CAD build for the part. Positions are in the model's coordinates, mm. A direction names the side the tool comes from. Give positions to 0.01 mm unless a question says otherwise; leave off trailing zeros. Order: outer loops, then holes, each group sorted by start corner. A loop starts at its lowest first (then second) coordinate and runs counter-clockwise, first axis right, second up.
Item 1: Band-saw the part on D-D on y = -13. Give the cut face in (x, z).
Item 2: Flat gauge pins, fed straight in: P1, Ø1.2, axis at y = -10.5, z = 2.5, coming from the -X side; P2, Ø2, axis at y = -8.5, z = 1.5, coming from the +X side; P3, Ø1.5, axis at x = -5, z = 1.5, coming from the -Y side. Where does each tip first touch, or does it go through?
Item 3: Band-saw the part on A-A on z = 0.9. Give the cut face in (x, y).
Item 4: Which spindle directions (+Z, -Z, +X, -X, +Y, -Y) get a long thin tool onto all of the face, cutting with end or side? Do faces 1 (the flat face through (2, -4, 0)), 2 (the flat face through (-2, -12, 2)), 3 (the flat face through (-2, 3, 2)). Say none if no direction does.
Item 5: Wall check: L1, parallel to X at y = -2, z = 2.55; L2, parallel to X at y = 5.25, z = 3.7; L3, parallel to X at y = -10, z = 3.4. Give the ranges that are in metal, low to high.
Item 6: Band-saw the part on B-B on y = 1. Give the cut face in (x, z).
Item 7: Two-plate mould, pull along X, no slides. Class faces 4 (the cylindrical face through (0, -5, 2)), 5 (the cylindrical face through (-8.1, -0.1, 2)), 6 (the flat face through (2, -12, 2)): released by +X, released by -X, zero draft, split by the parting line, or undercut.
Item 8: Band-saw the part on C-C on x = 0. Give the cut face in (y, z).
```python
from build123d import *

# Parameters (mm, degrees)
ESQUISSE1_W        = 4
ESQUISSE1_H        = 8
BOSS_EXTRU_1_DEPTH = 4


with BuildPart() as part:
    # Esquisse1 → Boss.-Extru.1 (new body)
    with BuildSketch(Plane.XY):
        with BuildLine():
            Line((-2, 7.849203781), (-2, -3))
            ThreePointArc((-2, -3), (0, -5), (2, -3))
            Line((2, -3), (2, 7.849203781))
            ThreePointArc((2, 7.849203781), (0, -8.1), (-2, 7.849203781))
        make_face()
        with Locations((0, -11.849203781)):
            Rectangle(ESQUISSE1_W, ESQUISSE1_H)
    extrude(amount=BOSS_EXTRU_1_DEPTH)


solid = part.part
```
The answers:
1. outline: (-2, 0) - (2, 0) - (2, 4) - (-2, 4) - close
2. P1: stops at x = -2
2. P2: stops at x = 3.06
2. P3: stops at y = -6.9
3. outline: (-2, -15.85) - (2, -15.85) - (2, -7.85) arc R8.1 ccw to (2, 7.85) - (2, -3) arc R2 cw to (-2, -3) - (-2, 7.85) arc R8.1 ccw to (-2, -7.85) - close
4. face 1: -Z, +X, -X, +Y, -Y
4. face 2: +Z, -Z, -X, -Y
4. face 3: +Z, -Z, +Y
5. L1: x = -7.85 to -2, 2 to 7.85
5. L2: x = -6.17 to -2, 2 to 6.17
5. L3: x = -2 to 2
6. outline: (-8.04, 0) - (-2, 0) - (-2, 4) - (-8.04, 4) - close; (2, 0) - (8.04, 0) - (8.04, 4) - (2, 4) - close
7. face 4: undercut
7. face 5: released by -X
7. face 6: released by +X
8. outline: (-15.85, 0) - (-5, 0) - (-5, 4) - (-15.85, 4) - close
